Input: dimensioned drawing with shaded views. Units: mm. Origin: part minimum x, y, z. A direction names the side the tool comes from. Give positions to 0.01 mm unless a question says otherwise; leave off trailing zeros. Loops run counter-clockwise (first coordinate to the right, second up) from the corner with the lowest first, then second, coordinate; pieces in that order, holes last. Notation, with made-up numbers: (46.5, 79.25) -> (94.5, 79.25) arc R25 ccw to (94.5, 104.25) -> close; hole circle Ø4 at (-4, -38.5). An arc over 180 degrees is marked (long way). Answer in a Markdown table with one row per item. Add a question column.
1) Section query C-C (z = 12.5). Return the cut outline in (x, y), plus the area to 3 significant figures.
2) Access query for the marked faces 1, 2, 3 and 4. Directions: +Z, -Z, +X, -X, +Y, -Y. A direction counts if a zero-diameter tool reaches every point of the face in a straight line with its end or side. Return the directions, or none.
3) First-contact query: P1, Ø4, axis at x = 37, y = 116.5, coming from the -Z side; P2, Ø12.5, axis at x = 82, z = 90, coming from the +Y side; P3, Ø4, axis at y = 46, z = 140.5, coming from the -X side. Flat tips, straight axial feed; report the tip coordinate or a pass-through.
4) Section query A-A (y = 85.5). Return the cut outline in (x, z), plus the area to 3 significant figures.
5) Line query: line 1 (Z direction, x = 4.5, y = 107.95); line 2 (Z direction, x = 59, y = 73); line 3 (Y direction, x = 82, z = 82). Output: solid intervals per line, ascending. Write a range as from..to.
6) Section query D-D (y = 44.45). Return the cut outline in (x, z).
7) Section query B-B (x = 45). Return the cut outline in (y, z), plus the area to 3 significant figures.
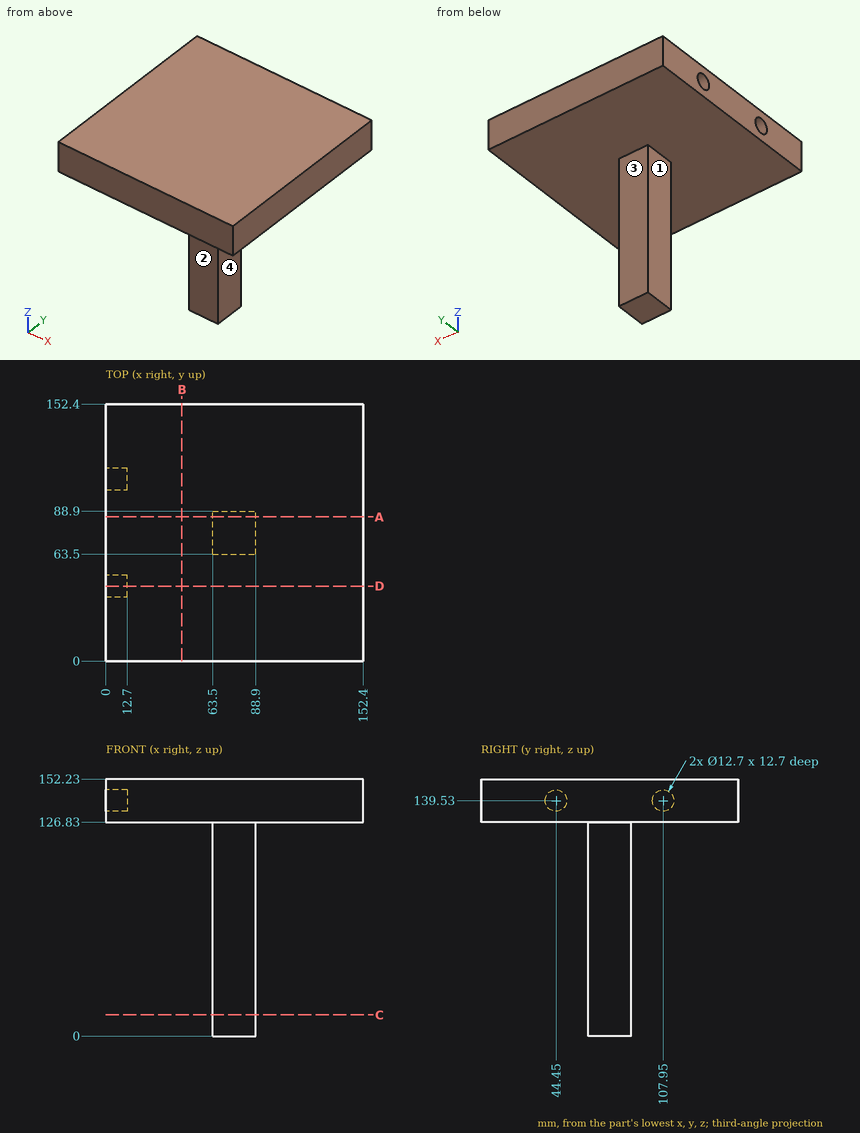
Evaluation:
| question | item | result |
|---|---|---|
| 1 | outline | (63.5, 63.5) -> (88.9, 63.5) -> (88.9, 88.9) -> (63.5, 88.9) -> close |
| 1 | area | 645 mm² |
| 2 | face 1 | -Z, -X, +Y, -Y |
| 2 | face 2 | -Z, +X, -X, -Y |
| 2 | face 3 | -Z, +X, -X, +Y |
| 2 | face 4 | -Z, +X, +Y, -Y |
| 3 | P1 | z = 126.83 |
| 3 | P2 | y = 88.9 |
| 3 | P3 | x = 12.7 |
| 4 | outline | (0, 126.83) -> (63.5, 126.83) -> (63.5, 0) -> (88.9, 0) -> (88.9, 126.83) -> (152.4, 126.83) -> (152.4, 152.23) -> (0, 152.23) -> close |
| 4 | area | 7,090 mm² |
| 5 | line 1 | 126.83..133.18, 145.88..152.23 |
| 5 | line 2 | 126.83..152.23 |
| 5 | line 3 | 63.5..88.9 |
| 6 | outline | (0, 126.83) -> (152.4, 126.83) -> (152.4, 152.23) -> (0, 152.23) -> (0, 145.88) -> (12.7, 145.88) -> (12.7, 133.18) -> (0, 133.18) -> close |
| 7 | outline | (0, 126.83) -> (152.4, 126.83) -> (152.4, 152.23) -> (0, 152.23) -> close |
| 7 | area | 3,870 mm² |
